Source: three-view drawing plus pictorial views. Frame: mm from the lowest corner of the part. A direction names the side the tool comes from. Coordinates: 2 decimals unless noted, no trailing zeros. Loops run counter-clockwise (first coordinate to the right, second up) from the corner with the lowest first, then second, coordinate; pieces in that order, holes last. Notation, with made-up numbers: (77.25, 13) - (94.25, 13) arc R18 cw to (94.25, 24) - close; hole circle Ø10 at (33.5, 24.25). An arc over 180 degrees is marked (long way). Return JSON: item names as keys, results as strings.
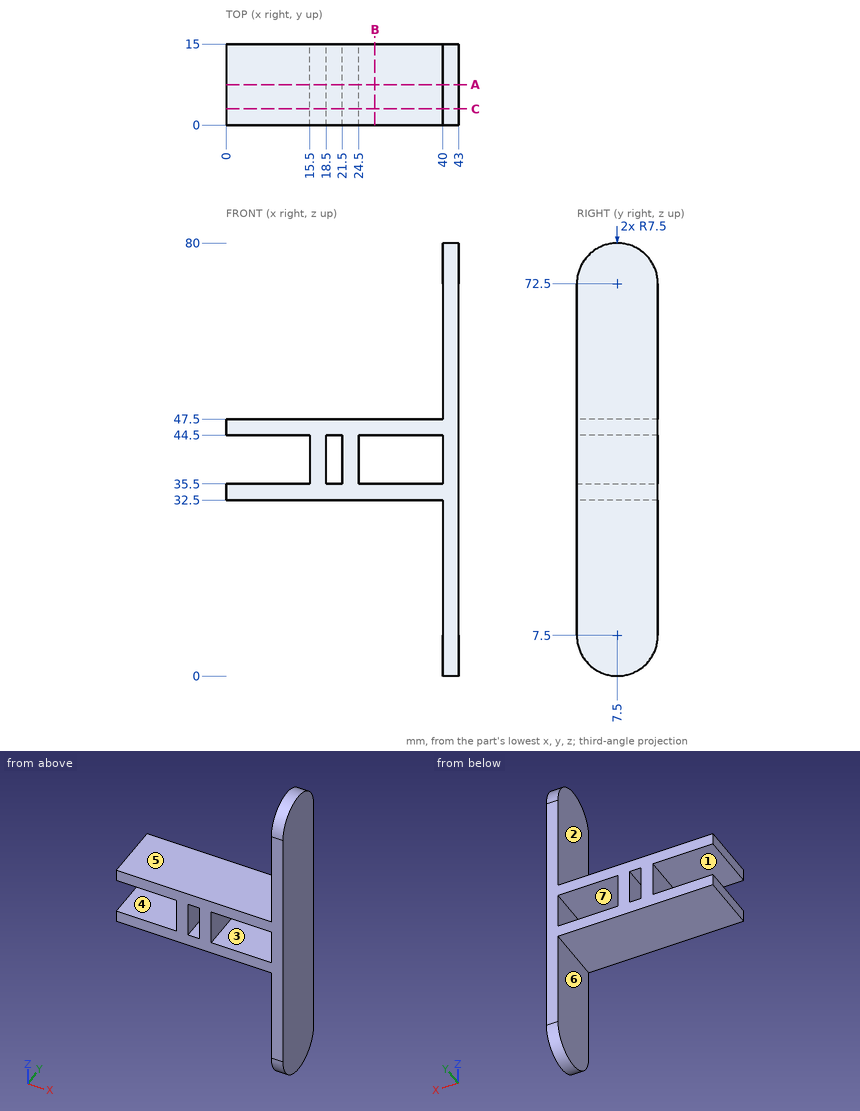
Item 1: Mould query, pull axis X, two halves, no side actions, for the marked faces 1, 2 and 3. Classes: +X half, -X half, draft (parallel to the pull), parting line (faces both ways), or undercut.
Worked out:
{"face 1": "draft", "face 2": "-X half", "face 3": "undercut"}
Item 2: First-contact query: pin 1 Ø7.5 at (y, z) = (4, 10.5) entering from -X; pin 2 Ø7.5 at (x, y) = (17.5, 11) entering from -Z; pin 3 Ø8 at (x, z) = (17, 49.5) entering from -Y; pin 4 Ø2 at (x, y) = (26.5, 11) entering from +Z. Flat tips, straight axial feed; report the tip coordinate or a pass-through.
Worked out:
{"pin 1": "x = 40", "pin 2": "z = 32.5", "pin 3": "y = 0", "pin 4": "z = 47.5"}
Item 3: Section query A-A, the plane y = 7.5. Return loops of the section in (x, z), and give its area (3 significant figures).
Worked out:
{"outline": "(0, 32.5) - (40, 32.5) - (40, 0) - (43, 0) - (43, 80) - (40, 80) - (40, 47.5) - (0, 47.5) - (0, 44.5) - (15.5, 44.5) - (15.5, 35.5) - (0, 35.5) - close; hole (18.5, 35.5) - (21.5, 35.5) - (21.5, 44.5) - (18.5, 44.5) - close; hole (24.5, 35.5) - (40, 35.5) - (40, 44.5) - (24.5, 44.5) - close", "area": "534 mm^2"}
Item 4: Reachability of the marked faces 4, 5, 6 and 7 from +Z, -Z, +X, -X, +Y, -Y: full face, straight path, thin tool, end or side. Return the list, or none.
Worked out:
{"face 4": "-X, +Y, -Y", "face 5": "+Z, -X, +Y, -Y", "face 6": "-Z, -X, +Y, -Y", "face 7": "+Y, -Y"}
Item 5: Section query C-C, the plane y = 3. Return loops of the section in (x, z).
Worked out:
{"outline": "(0, 32.5) - (40, 32.5) - (40, 1.5) - (43, 1.5) - (43, 78.5) - (40, 78.5) - (40, 47.5) - (0, 47.5) - (0, 44.5) - (15.5, 44.5) - (15.5, 35.5) - (0, 35.5) - close; hole (18.5, 35.5) - (21.5, 35.5) - (21.5, 44.5) - (18.5, 44.5) - close; hole (24.5, 35.5) - (40, 35.5) - (40, 44.5) - (24.5, 44.5) - close"}
Item 6: Ray query, probe 1 along X at (y, z) = (7.75, 43.5); probe 2 along Z at (x, y) = (29, 7.75); probe 3 along X at (y, z) = (5, 75). Return the intervals inside material, ascending. Write a range as from..to.
Worked out:
{"probe 1": "15.5..18.5, 21.5..24.5, 40..43", "probe 2": "32.5..35.5, 44.5..47.5", "probe 3": "40..43"}
Item 7: Section query B-B, the plane x = 27.5. Return loops of the section in (y, z).
Worked out:
{"outline": "(0, 32.5) - (15, 32.5) - (15, 35.5) - (0, 35.5) - close; (0, 44.5) - (15, 44.5) - (15, 47.5) - (0, 47.5) - close"}
